Check sheet for the modelled part. Datum: model origin and axes. Units: mm. Give positions to 0.01 mm unless a question says otherwise; leave off trailing zeros. Loops run counter-clockwise (first coordinate to the right, second up) from the corner with the lowest first, then second, coordinate; pieces in that order, holes last. Notation, with made-up numbers: (6.25, 33.5) - (48.25, 33.5) arc R9 cw to (48.25, 49.5) - close; hole circle Ø10 at (36.25, 86.25). An arc over 180 degrees is marked (long way). Answer in a Markdown table with one row per item. Add a question column.
(1) Go/stop test with flat-tipped pins: P1, Ø3, axis at x = -76.64, z = 66.07, coming from the -Y side; P2, Ø1.5, axis at x = -23.5, y = 1.5, coming from the -Z side; P3, Ø1, axis at x = -33, y = 0.5, coming from the -Z side; P4, Ø1, axis at x = 23, y = 2, coming from the -Z side. Record where each tip stops, or that it passes through.
(2) Thickness scan on L1, parallel to X at y = 2.5, z = 65; L2, parallel to Z at x = 58, y = 1.8; L3, parallel to Z at x = 68, y = 2.65. Record the ranges inside material, lowest first.
(3) Sectioned sample at A-A on x = -4.5. Enter the section's corners in (y, z), then the cut area to 3 significant figures.
(4) Sectioned sample at B-B on y = 1.1. State how many separate pieces and enclosed holes the cut face has, then the cut area to 3 significant figures.
from build123d import *

# Parameters (mm, degrees)
BOSS_EXTRUDE1_DEPTH = 3
BOSS_EXTRUDE2_DEPTH = 2
SKETCH6_R           = 2.6
CUT_EXTRUDE6_DEPTH  = 167.076115532
SKETCH3_R           = 2.6
CUT_EXTRUDE7_DEPTH  = 167.076115532
CUT_EXTRUDE8_DEPTH  = 167.076115532


with BuildPart() as part:
    # Sketch1 → Boss-Extrude1 (new body)
    with BuildSketch(Plane(origin=(0, 0, 0), x_dir=(1, 0, 0), z_dir=(0, 1, 0))):
        Polygon((-59.316686906, 108.225499677), (101.185838411, 108.225499677), (125.934575753, 83.476762335), (125.934575753, -77.025762982), (101.185838411, -101.774500323), (-59.316686906, -101.774500323), (-84.065424247, -77.025762982), (-84.065424247, 83.476762335), align=None)
    extrude(amount=BOSS_EXTRUDE1_DEPTH)

    # Sketch2 → Boss-Extrude2 (add)
    with BuildSketch(Plane(origin=(0, 3, 0), x_dir=(1, 0, 0), z_dir=(0, 1, 0))):
        Polygon((-84.065424247, -77.025762982), (-45.174551282, -38.134890016), (-20.425813941, -62.883627358), (-59.316686906, -101.774500323), align=None)
        Polygon((125.934575753, -77.025762982), (93.880849872, -37.104770943), (66.751068905, -58.888061335), (101.185838411, -101.774500323), align=None)
        Polygon((101.185838411, 108.225499677), (62.16108336, 69.955487183), (86.665825958, 44.96747398), (125.934575753, 83.476762335), align=None)
        Polygon((-59.316686906, 108.225499677), (-24.100270952, 65.978558399), (-50.874640527, 43.659845911), (-84.065424247, 83.476762335), align=None)
    extrude(amount=-BOSS_EXTRUDE2_DEPTH)

    # Sketch6 → Cut-Extrude6 (cut, through all)
    with BuildSketch(Plane(origin=(0, 3, 0), x_dir=(1, 0, 0), z_dir=(0, 1, 0))):
        with Locations(Location((-18.065424247, 52.225499677, 0), (0, 0, 270))):
            Circle(SKETCH6_R)
        with Locations(Location((59.934575753, 52.225499677, 0), (0, 0, 270))):
            Circle(SKETCH6_R)
        with Locations(Location((59.934575753, -45.774500323, 0), (0, 0, 270))):
            Circle(SKETCH6_R)
        with Locations(Location((-18.065424247, -45.774500323, 0), (0, 0, 270))):
            Circle(SKETCH6_R)
        with Locations(Location((20.934575753, -45.774500323, 0), (0, 0, 270))):
            Circle(SKETCH6_R)
        with Locations(Location((20.934575753, 52.225499677, 0), (0, 0, 270))):
            Circle(SKETCH6_R)
    extrude(amount=-CUT_EXTRUDE6_DEPTH, mode=Mode.SUBTRACT)

    # Sketch3 → Cut-Extrude7 (cut, through all)
    with BuildSketch(Plane(origin=(0, 3, 0), x_dir=(1, 0, 0), z_dir=(0, 1, 0))):
        with Locations(Location((-27.143328362, 79.587675039, 0), (0, 0, 270))):
            Circle(SKETCH3_R)
        with Locations(Location((-55.427599609, 51.303403791, 0), (0, 0, 270))):
            Circle(SKETCH3_R)
        with Locations(Location((-76.640803045, 72.516607227, 0), (0, 0, 270))):
            Circle(SKETCH3_R)
        with Locations(Location((-48.356531798, 100.800878474, 0), (0, 0, 270))):
            Circle(SKETCH3_R)
        with Locations(Location((118.50995455, 72.516607227, 0), (0, 0, 90))):
            Circle(SKETCH3_R)
        with Locations(Location((97.296751114, 51.303403791, 0), (0, 0, 90))):
            Circle(SKETCH3_R)
        with Locations(Location((69.012479867, 79.587675039, 0), (0, 0, 90))):
            Circle(SKETCH3_R)
        with Locations(Location((90.225683303, 100.800878474, 0), (0, 0, 90))):
            Circle(SKETCH3_R)
        with Locations(Location((-55.427599609, -44.852404438, 0), (0, 0, 90))):
            Circle(SKETCH3_R)
        with Locations(Location((-76.640803045, -66.065607873, 0), (0, 0, 90))):
            Circle(SKETCH3_R)
        with Locations(Location((-48.356531798, -94.349879121, 0), (0, 0, 90))):
            Circle(SKETCH3_R)
        with Locations(Location((-27.143328362, -73.136675685, 0), (0, 0, 90))):
            Circle(SKETCH3_R)
        with Locations(Location((118.50995455, -66.065607873, 0), (0, 0, 270))):
            Circle(SKETCH3_R)
        with Locations(Location((97.296751114, -44.852404438, 0), (0, 0, 270))):
            Circle(SKETCH3_R)
        with Locations(Location((90.225683303, -94.349879121, 0), (0, 0, 270))):
            Circle(SKETCH3_R)
        with Locations(Location((69.012479867, -73.136675685, 0), (0, 0, 270))):
            Circle(SKETCH3_R)
    extrude(amount=-CUT_EXTRUDE7_DEPTH, mode=Mode.SUBTRACT)

    # Sketch7 → Cut-Extrude8 (cut, through all)
    with BuildSketch(Plane(origin=(0, 3, 0), x_dir=(1, 0, 0), z_dir=(0, 1, 0))):
        Polygon((-14.065424247, 83.225499677), (55.934575753, 83.225499677), (80.934575753, 108.225499677), (-39.065424247, 108.225499677), align=None)
        Polygon((-14.065424247, -76.774500323), (-39.065424247, -101.774500323), (80.934575753, -101.774500323), (55.934575753, -76.774500323), align=None)
    extrude(amount=-CUT_EXTRUDE8_DEPTH, mode=Mode.SUBTRACT)


solid = part.part
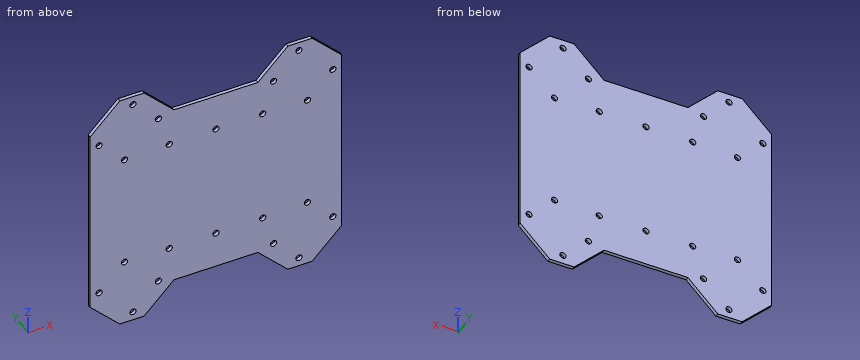
Reply:
| question | item | result |
|---|---|---|
| 1 | P1 | through |
| 1 | P2 | z = -93.41 |
| 1 | P3 | z = -102.66 |
| 1 | P4 | z = -83.23 |
| 2 | L1 | -84.07 to -79.01, -74.27 to 116.14, 120.88 to 125.93 |
| 2 | L2 | -85.29 to -53.96, -50.49 to 44.04, 47.51 to 78.84 |
| 2 | L3 | -95.29 to -81.98, -77.19 to 70.74, 75.53 to 88.84 |
| 3 | outline | (0, -83.23) - (3, -83.23) - (3, 76.77) - (0, 76.77) - close |
| 3 | area | 480 mm^2 |
| 4 | separate pieces | 1 |
| 4 | enclosed holes | 22 |
| 4 | area | 37,700 mm^2 |
